Design review of the part built by this model. Coordinates are the model's own, in mm. A direction names the side the tool comes from. Give positions to 0.01 mm unless a question says otherwise; leave off trailing zeros. Loops run counter-clockwise (first coordinate to the right, second up) from the corner with the lowest first, then second, coordinate; pieces in that order, holes last. Notation, with made-up numbers: (71.5, 81) - (80.5, 81) arc R14 cw to (80.5, 89) - close; hole circle Ø3 at (-25, -10.5). An arc over 180 degrees is marked (long way). Put each result on its own line as item: value. Start each with the question number.
```python
from build123d import *

# Parameters (mm, degrees)
BASPROSKE_W        = 12
BASPROSKE_H        = 22
TOOTHCUT_DEPTH     = 34.346664001
TEETHCUTS_COUNT    = 20
TEETHCUTS_ANGLE    = 342
BORSKE_R           = 1.5
BORE_DEPTH         = 50.0000508
SKETCH1_R          = 0.75
CUT_EXTRUDE1_DEPTH = 12
CUT_EXTRUDE2_DEPTH = 3
CIRPATTERN1_COUNT  = 4


with BuildPart() as part:
    # BasProSke → Base-Revolve (revolve)
    with BuildSketch(Plane(origin=(0, 0, 0), x_dir=(1, 0, 0), z_dir=(0, 1, 0)), mode=Mode.PRIVATE) as base_revolve_sk:
        with Locations((6, 11)):
            Rectangle(BASPROSKE_W, BASPROSKE_H)
    revolve(base_revolve_sk.sketch.rotate(Axis((-10, 0, 0), (1, 0, 0)), 180), axis=Axis((-10, 0, 0), (1, 0, 0)))

    # TooCutSke → ToothCut (cut, through all)
    with BuildSketch(Plane(origin=(0, 0, 0), x_dir=(0, 0, -1), z_dir=(1, 0, 0))):
        with BuildLine():
            ThreePointArc((0.986171591, 17.471189616), (0, 17.499), (-0.986171591, 17.471189616))
            ThreePointArc((-0.986171591, 17.471189616), (-1.626916196, 19.798789858), (-2.932850173, 21.829260982))
            ThreePointArc((-2.932850173, 21.829260982), (0, 22.0254), (2.932850173, 21.829260982))
            ThreePointArc((2.932850173, 21.829260982), (1.626916196, 19.798789858), (0.986171591, 17.471189616))
        make_face()
    toothcut = extrude(amount=TOOTHCUT_DEPTH, mode=Mode.SUBTRACT)

    # TeethCuts: ToothCut ×20 about axis
    teethcuts_axis = Axis((-10, 0, 0), (1, 0, 0))
    for i in range(1, TEETHCUTS_COUNT):
        add(toothcut.rotate(teethcuts_axis, i * TEETHCUTS_ANGLE / (TEETHCUTS_COUNT - 1)), mode=Mode.SUBTRACT)

    # BorSke → Bore (cut, symmetric)
    with BuildSketch(Plane(origin=(0, 0, 0), x_dir=(0, 0, -1), z_dir=(1, 0, 0))):
        with Locations(Location((0, 0, 0), (0, 0, 180))):
            Circle(BORSKE_R)
    extrude(amount=BORE_DEPTH, both=True, mode=Mode.SUBTRACT)

    # Sketch1 → Cut-Extrude1 (cut)
    with BuildSketch(Plane(origin=(12, 0, 0), x_dir=(0, 0, -1), z_dir=(1, 0, 0))):
        with Locations((-3.356833967, 13.075995783)):
            Circle(SKETCH1_R)
        with Locations((-2.610870863, 10.170218942)):
            Circle(SKETCH1_R)
        with Locations((10.170218942, 2.610870863)):
            Circle(SKETCH1_R)
        with Locations((13.075995783, 3.356833967)):
            Circle(SKETCH1_R)
        with Locations((-7.264442102, -1.864907759)):
            Circle(SKETCH1_R)
        with Locations((-10.170218942, -2.610870863)):
            Circle(SKETCH1_R)
        with Locations((1.864907759, -7.264442102)):
            Circle(SKETCH1_R)
        with Locations((3.356833967, -13.075995783)):
            Circle(SKETCH1_R)
        with Locations((-1.864907759, 7.264442102)):
            Circle(SKETCH1_R)
        with Locations((7.264442102, 1.864907759)):
            Circle(SKETCH1_R)
        with Locations((-13.075995783, -3.356833967)):
            Circle(SKETCH1_R)
        with Locations((2.610870863, -10.170218942)):
            Circle(SKETCH1_R)
    extrude(amount=-CUT_EXTRUDE1_DEPTH, mode=Mode.SUBTRACT)

    # Sketch1<3> → Cut-Extrude2 (cut)
    with BuildSketch(Plane(origin=(12, 0, 0), x_dir=(0, 0, -1), z_dir=(1, 0, 0))):
        with BuildLine():
            Line((-2.460152648, 8.677810145), (-2.447111692, 8.646845292))
            ThreePointArc((-2.447111692, 8.646845292), (-1.491875211, 5.811566774), (-2.020691692, 8.756330625))
            Line((-2.020691692, 8.756330625), (-2.033064445, 8.785971947))
            ThreePointArc((-2.033064445, 8.785971947), (-1.150777462, 10.513915407), (-2.71120657, 11.666859429))
            ThreePointArc((-2.71120657, 11.666859429), (-3.742248237, 14.577313817), (-3.24385833, 11.530118522))
            ThreePointArc((-3.24385833, 11.530118522), (-4.057266963, 9.772804395), (-2.460152648, 8.677810145))
        make_face()
    cut_extrude2 = extrude(amount=-CUT_EXTRUDE2_DEPTH, mode=Mode.SUBTRACT)

    # CirPattern1: Cut-Extrude2 ×4 about axis
    cirpattern1_axis = Axis((0, 0, 0), (1, 0, 0))
    for i in range(1, CIRPATTERN1_COUNT):
        add(cut_extrude2.rotate(cirpattern1_axis, i * 360 / CIRPATTERN1_COUNT), mode=Mode.SUBTRACT)


solid = part.part
```
Item 1: Consider section A-A (z = 13). State the section outline as (x, y) points, plus the area to 3 significant figures.
Item 2: For P1, Ø2, axis at y = -1.86, z = 7.26, coming from the +X side; P2, Ø1.5, axis at x = 2, y = -4, coming from the +Z side; P3, Ø6, axis at x = 2.5, y = -6.5, coming from the +Z side, all flat-tipped, find the tip position at first contact; note any pin that passes through.
Item 3: For L1, parallel to Z at x = 1.5, y = 3; L2, parallel to Z at x = 10.5, y = -17; L3, parallel to Y at x = 1, z = 15.5, list the stretches that pass through material, from the lowest coordinate up. Write a range as from..to.
Item 4: Mouldability with a two-part tool opening along Y and no side actions: class faces 1 (the cylindrical face through (10.52, -14.59, -3.68)), 2 (the cylindrical face through (6.084, -21.728, 3.449)), 3 (the cylindrical face through (5.92, 18.29, 7.63)) as pulls with the +Y half, pulls with the -Y half, needs draft (parallel to the pull), parting line crosses it, or undercut.
Item 5: Consider section B-B (x = 4). Count the separate pieces of the cut face and the enclosed holes in it, plus the area to 3 significant figures.
Item 6: Machinability: for faces 4 (the cylindrical face through (5.92, -15.07, 12.97)), 5 (the cylindrical face through (5.92, 7.63, -18.29)), 6 (the cylindrical face through (10.521, 1.553, -5.797)), 7 (the cylindrical face through (5.916, -19.284, 4.576)), which of the approach directions +Z, -Z, +X, -X, +Y, -Y give a long, thin tool a straight path to every point of the face, cutting with its end or side? Answer none if there is none.
Geometry says:
1. outline: (0, -15.09) - (12, -15.09) - (12, -4.9) - (9, -4.9) - (9, -4.1) - (0, -4.1) - close; (0, -2.61) - (9, -2.61) - (9, -1.81) - (12, -1.81) - (12, 15.09) - (0, 15.09) - close
1. area: 339 mm2
2. P1: stops at x = 9
2. P2: stops at z = 21.76
2. P3: stops at z = 21.72
3. L1: z = -21.79..-13.74, -12.42..-10.81, -9.53..21.79
3. L2: z = -10.33..-6.7, -4.48..4.48, 6.7..10.33
3. L3: y = -15.61..-13.84, -9.86..9.86, 13.84..15.61
4. face 1: undercut
4. face 2: pulls with the -Y half
4. face 3: pulls with the +Y half
5. separate pieces: 1
5. enclosed holes: 13
5. area: 1,190 mm2
6. face 4: +X, -X, -Y
6. face 5: -Z, +X, -X
6. face 6: +X
6. face 7: +X, -X
